Work out the finished part from the listing and answer in its coordinate system (mm). Face numbers are marked on the shaded views. A direction names the side the tool comes from. Round coordinates to 2 decimals unless told otherwise and drop trailing zeros. Order: outer loops, then holes, each group sorted by start corner. A loop starts at its lowest first (then second) coordinate and runs counter-clockwise, first axis right, second up. Notation, with made-up numbers: M -30,69.5 L 29,69.5 A36 cw 29,105.5 Z; hole C 83,20 d5. An arc over 180 degrees is marked long. Return JSON: item names as keys, results as strings.
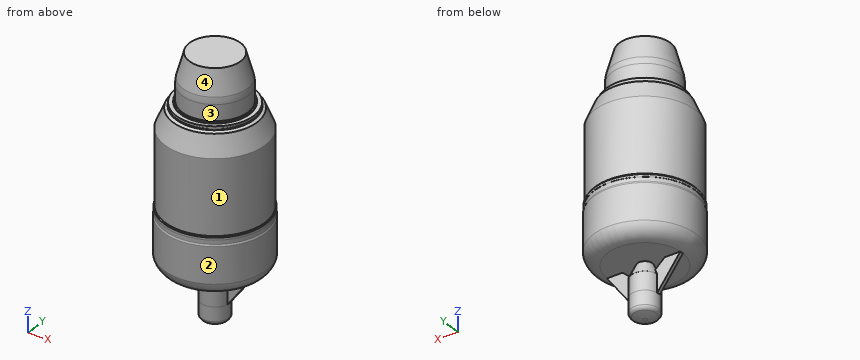
Autodesk Inventor part; units mm, degrees
ref_plane "YZ Plane" through (0, 0, 0) normal (1, 0, 0) x (0, 1, 0)
ref_plane "XZ Plane" through (0, 0, 0) normal (0, 1, 0) x (-1, 0, 0)
ref_plane "XY Plane" through (0, 0, 0) normal (0, 0, 1) x (1, 0, 0)
sketch "Sketch3" plane through (0, 0, 0) normal (0, 1, 0) x (-1, 0, 0)
  line L0 (-148.4998, -210.0502) -> (-148.4998, 210.0502) construction
  line L1 (-148.4998, 210.0502) -> (148.4998, 210.0502) construction
  line L2 (148.4998, 210.0502) -> (148.4998, -210.0502) construction
  line L3 (148.4998, -210.0502) -> (-148.4998, -210.0502) construction
  line L4 (-278.8232, 0) -> (0, 0) construction
  line L5 (0, 0) -> (0, 323.3607) construction
  line L6 (-14.9991, -133.5139) -> (-14.9991, -118.3294)
  line L7 (-56, -69.6027) -> (-56, -30.1317)
  line L8 (-56, -30.1317) -> (-55.287, -28.2144)
  line L9 (-55.287, -28.2144) -> (-55.287, -23.6926)
  line L10 (-55.287, -23.6926) -> (-55.4718, -23.6926)
  line L11 (-55.4718, -23.6926) -> (-55.4718, -20.982)
  line L12 (-55.4718, -20.982) -> (-54.6709, -19.7868)
  line L13 (-54.6709, -19.7868) -> (-54.6709, 61.4098)
  line L14 (-54.6709, 61.4098) -> (-45.8766, 82.3346)
  line L15 (-45.8766, 82.3346) -> (-42.7179, 84.1079)
  line L16 (-42.7179, 84.1079) -> (-42.7179, 85.2162)
  line L17 (-42.7179, 85.2162) -> (-42.369, 85.2162)
  line L18 (-42.369, 85.2162) -> (-42.369, 88.0675)
  line L19 (-42.369, 88.0675) -> (-37.697, 88.0675)
  line L20 (-37.697, 88.0675) -> (-37.697, 89.6261)
  line L21 (-37.697, 89.6261) -> (-35.994, 89.6261)
  line L22 (-35.994, 89.6261) -> (-35.994, 106.9741)
  line L23 (-35.3011, 114.3761) -> (-28.055, 140.5061)
  line L24 (-28.055, 140.5061) -> (0, 140.5061)
  arc A0 (-12.1858, -137.6578) -> (-2.3721, -140.4939) centre (-0.8223, -116.7339) ccw
  arc A1 (-14.9991, -133.5139) -> (-12.1858, -137.6578) centre (-9.5817, -132.8629) ccw
  line L25 (0, -140.4939) -> (-2.3721, -140.4939)
  line L26 (0, 140.5061) -> (0, -140.4939)
  arc A2 (-35.3011, 114.3761) -> (-35.994, 106.9741) centre (-5.1555, 107.8209) ccw
  arc A3 (-56, -69.6027) -> (-40.4601, -83.9729) centre (-39.3408, -67.175) ccw
  line L27 (-40.4601, -83.9729) -> (-8.2198, -83.9729)
  line L28 (-8.2198, -83.9729) -> (-14.9991, -98.5086)
  line L29 (-14.9991, -98.5086) -> (-14.9991, -118.3294)
  dimension "d79" = 281
  dimension "d83" = 56
revolve "Motor" add sketch "Sketch3" angle 360 about axis through (0, 0, 140.5061) along (0, 0, -1)
sketch "Sketch6" plane through (0, 0, 0) normal (0, 1, 0) x (-1, 0, 0)
  line L0 (-14.9991, -118.4458) -> (-14.9991, -98.5086)
  line L1 (-12.6573, -93.4875) -> (-23.2868, -83.9729)
  line L2 (-23.2868, -83.9729) -> (-40.5228, -83.9729)
  line L3 (-40.5228, -83.9729) -> (-14.9991, -118.4458)
  line L4 (14.9991, -98.5086) -> (-14.9991, -98.5086)
  line L5 (-14.9991, -98.5086) -> (-12.6573, -93.4875)
  line L6 (0, -142.1349) -> (0, 23.6892) construction
  line L7 (14.9991, -118.4458) -> (14.9991, -98.5086)
  line L8 (12.6573, -93.4875) -> (23.2868, -83.9729)
  line L9 (23.2868, -83.9729) -> (40.5228, -83.9729)
  line L10 (40.5228, -83.9729) -> (14.9991, -118.4458)
  line L11 (14.9991, -98.5086) -> (12.6573, -93.4875)
  point P0 (0, 0)
extrude "Motor inlet" add sketch "Sketch6" along normal mid plane 4
properties part number "Engine"
Item 1: Consider line 1 along Z through (x, y) = (-2, 24.5); line 2 along Y through (x, z) = (22, -108); line 3 along Y through (x, z) = (0, -28). Determine where each line is inside the solid, lowest interval first. Write a range as [from, to].
Output:
{"line 1": "z = [-83.97, 140.51]", "line 2": "y = [-2, 2]", "line 3": "y = [-55.29, 55.29]"}
Item 2: Find section C-C (z = 53.5). Determine the outline of the cut face in (x, y).
Output:
{"outline": "C 0,0 d109.34"}
Item 3: Find section A-A (z = -89.5). Determine the outline of the cut face in (x, y), plus the area to 3 significant figures.
Output:
{"outline": "M -36.43,-2 L -17.11,-2 L -17.11,2 L -36.43,2 Z; C 0,0 d21.6; M 17.11,-2 L 36.43,-2 L 36.43,2 L 17.11,2 Z", "area": "521 mm^2"}
Item 4: Which of the six approach directions +Z, -Z, +X, -X, +Y, -Y give full straight-line access (tool end or side, diameter ignored) to the marked faces 1 and 2?
Output:
{"face 1": "+Z", "face 2": "+Z, -Z"}
Item 5: The mould has two halves that part along Z. Classify the marked faces 3 and 4: pulls with the +Z half, pulls with the -Z half, needs draft (parallel to the pull), parting line crosses it, or undercut.
Output:
{"face 3": "needs draft", "face 4": "pulls with the +Z half"}
Item 6: Each of these flat-tipped pins is pushed along its axis until it touches: pin 1 (2 mm diameter, centred on y = 1, z = -108, fed in from +X); pin 2 (8.5 mm diameter, centred on x = 21, z = -98.5, fed in from +Y); pin 3 (1 mm diameter, centred on y = 1, z = -108, fed in from -X). Where does it stop, or does it pass through?
Output:
{"pin 1": "stops at x = 23.47", "pin 2": "stops at y = 2", "pin 3": "stops at x = -23.1"}
Item 7: Find section B-B (z = -38.5). Determine the outline of the cut face in (x, y).
Output:
{"outline": "C 0,0 d112"}
